Could you check a few things on this drawing? It's one solid part, dimensions in mm from its lowest x, y, z. A direction names the side the tool comes from. Coordinates: 2 decimals unless noted, no trailing zeros. Write each loop counter-clockwise with the first axis right and the second up, starting at its lowest first coordinate (ties: lowest second). Pieces come first, ordered by that corner, then holes.
Item 1: For the marked faces 1 and 2, which set-ups out of +Z, -Z, +X, -X, +Y, -Y let a thin tool reach every point of the face, with its end or its side?
Item 2: If we mould it in two halves opening along Z, with no side actions, what happens to the marked faces 3, 4 and 5? For each: pulls with the +Z half, pulls with the -Z half, needs draft (parallel to the pull), parting line crosses it, or undercut.
Item 3: I want a section at A-A (x = 28). Please give me the cut outline in (y, z) (1 decimal).
Item 4: I'm going to push flat-ended pins straight in: P1, Ø3, axis at y = 21.5, z = 13.5, coming from the -X side (1 decimal); P2, Ø3, axis at x = 45, z = 21, coming from the +Y side; P3, Ø12, axis at x = 24.5, z = 48, coming from the -Y side. Where does each tip first touch, or does it pass through?
Item 5: I want a section at B-B (y = 20.25). Please give me the cut outline in (x, z) (1 decimal), and give its area (3 significant figures).
Item 6: I want a section at C-C (y = 9.25). Please give me the cut outline in (x, z) (1 decimal).
Item 7: Please list where these lines run through material, in increasing order: line 1 (X direction, y = 12.3, z = 28); line 2 (X direction, y = 18.25, z = 8.5).
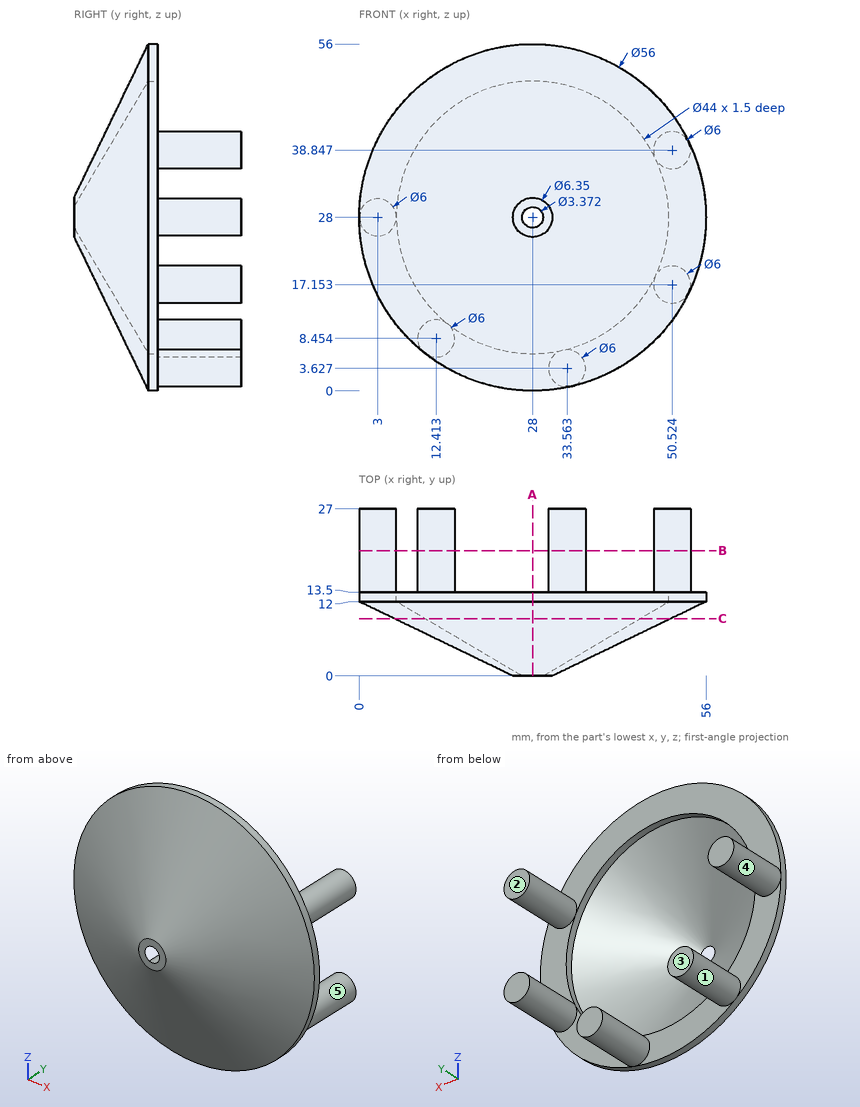
Answer:
1. face 1: +Y
1. face 2: +Z, -Z, +X, -X, +Y
2. face 3: needs draft
2. face 4: parting line crosses it
2. face 5: undercut
3. outline: (0, 24.8) - (12, 0) - (13.5, 0) - (13.5, 6) - (12, 6) - (0, 26.3) - close; (0, 29.7) - (12, 50) - (13.5, 50) - (13.5, 56) - (12, 56) - (0, 31.2) - close
4. P1: stops at x = 48.4
4. P2: stops at y = 10.75
4. P3: stops at y = 5.38
5. outline: circle Ø6 at (3, 28); circle Ø6 at (12.4, 8.5); circle Ø6 at (33.6, 3.6); circle Ø6 at (50.5, 17.2); circle Ø6 at (50.5, 38.8)
5. area: 141 mm2
6. outline: circle Ø44.6 at (28, 28); hole circle Ø34.7 at (28, 28)
7. line 1: x = 0 to 6, 50 to 56
7. line 2: x = 9.41 to 15.41
